from build123d import *

# Parameters (mm, degrees)
SKETCH_1_R          = 6.05
SKETCH_1_R_2        = 2.5
EXTRUDE_1_DEPTH     = 7.4
SKETCH_2_R          = 9
EXTRUDE_2_DEPTH     = 0.6
EXTRUDE_START       = -0.6
SKETCH_3_R          = 9
EXTRUDE_3_DEPTH     = 0.6
SKETCH_4_R          = 2.5
CUT_EXTRUDE_1_DEPTH = 15.722771478


with BuildPart() as part:
    # Эскиз1 → Бобышка-Вытянуть1 (new body)
    with BuildSketch(Plane.XY):
        Circle(SKETCH_1_R)
        Circle(SKETCH_1_R_2, mode=Mode.SUBTRACT)
    extrude(amount=EXTRUDE_1_DEPTH)

    # Эскиз2 → Бобышка-Вытянуть2 (add)
    with BuildSketch(Plane.XY.offset(7.4)):
        Circle(SKETCH_2_R)
    extrude(amount=-EXTRUDE_2_DEPTH)

    # Эскиз3 → Бобышка-Вытянуть3 (add)
    with BuildSketch(Plane(origin=(0, 0, 0), x_dir=(-1, 0, 0), z_dir=(0, 0, -1)).offset(EXTRUDE_START)):
        with Locations(Location((0, 0, 0), (0, 0, 180))):
            Circle(SKETCH_3_R)
    extrude(amount=EXTRUDE_3_DEPTH)

    # Эскиз4 → Вырез-Вытянуть1 (cut, through all)
    with BuildSketch(Plane.XY.offset(7.4)):
        Circle(SKETCH_4_R)
    extrude(amount=-CUT_EXTRUDE_1_DEPTH, mode=Mode.SUBTRACT)


solid = part.part
The model under review builds one solid part; all positions refer to its coordinate system, in mm. A direction names the side the tool comes from. Round coordinates to 2 decimals unless told otherwise and drop trailing zeros. Order: outer loops, then holes, each group sorted by start corner. A loop starts at its lowest first (then second) coordinate and runs counter-clockwise, first axis right, second up. Notation, with made-up numbers: (52, 26) -> (69, 26) arc R36 cw to (69, 62) -> close; hole circle Ø11 at (42, 83.5). An arc over 180 degrees is marked (long way). Return JSON: item names as keys, results as strings.
1. Take a section at D-D (x = 7.5). Write out the cut boundary in (y, z).
Answer block:
{"outline": "(-4.97, 0) -> (4.97, 0) -> (4.97, 0.6) -> (-4.97, 0.6) -> close; (-4.97, 6.8) -> (4.97, 6.8) -> (4.97, 7.4) -> (-4.97, 7.4) -> close"}
2. Insertion check: P1, Ø1.5, axis at y = 0.5, z = 3, coming from the -X side; P2, Ø1, axis at y = -4, z = 6, coming from the -X side; P3, Ø4, axis at x = 0, y = 0, coming from the -Z side; P4, Ø1, axis at x = 0, z = 1.5, coming from the -Y side. Each pin has a flat end and moves straight along its axis. Give the tip position at first contact, or say it passes through.
Answer block:
{"P1": "stops at x = -6.05", "P2": "stops at x = -4.93", "P3": "passes through", "P4": "stops at y = -6.05"}
3. Take a section at A-A (y = 0). Write out the cut boundary in (x, z), then the cut area to 3 significant figures.
Answer block:
{"outline": "(-9, 0) -> (-2.5, 0) -> (-2.5, 7.4) -> (-9, 7.4) -> (-9, 6.8) -> (-6.05, 6.8) -> (-6.05, 0.6) -> (-9, 0.6) -> close; (2.5, 0) -> (9, 0) -> (9, 0.6) -> (6.05, 0.6) -> (6.05, 6.8) -> (9, 6.8) -> (9, 7.4) -> (2.5, 7.4) -> close", "area": "59.6 mm²"}
4. Take a section at C-C (z = 5.75). Write out the cut boundary in (x, y).
Answer block:
{"outline": "circle Ø12.1 at (0, 0); hole circle Ø5 at (0, 0)"}
5. The part is to be moulded in two halves that separate along Y. For faces 3 (the face through (2, 6, 0.6)), 4 (the face through (-0.54, -2.44, 3.75)), 5 (the face through (5.589, -2.317, 3.657)), say which applies: +Y half, -Y half, draft (parallel to the pull), parting line (faces both ways), or undercut.
Answer block:
{"face 3": "draft", "face 4": "undercut", "face 5": "parting line"}
6. For L1, parallel to Y at x = 0, z = 6; L2, parallel to Z at x = 7.5, y = 4.75; L3, parallel to X at y = 0.75, z = 0.75, list the stretches that pass through material, from the lowest coordinate up. Write a range as [from, to].
Answer block:
{"L1": "y = [-6.05, -2.5], [2.5, 6.05]", "L2": "z = [0, 0.6], [6.8, 7.4]", "L3": "x = [-6, -2.38], [2.38, 6]"}
7. For faces 1 (the face through (2, -6, 6.8)), 2 (the face through (-6.633, -6.083, 0.304)), list the 3-axis set-ups (+Z, -Z, +X, -X, +Y, -Y) from which the entire face can be reached by the end or side of a thin tool; tool diameter is ignored.
Answer block:
{"face 1": "none", "face 2": "+Z, -Z"}
